```python
from build123d import *

# Parameters (mm, degrees)
SKETCH2_R         = 0.8
SKETCH4_R         = 0.9
EXTRUDE1_DEPTH    = 6
SKETCH5_OUTSIDE_W = 12.282
SKETCH5_OUTSIDE_H = 20.656
SKETCH5_OUTSIDE_R = 0.75
EXTRUDE3_DEPTH    = 11


with BuildPart() as part:
    # Sweep1: sweep along a path in Sketch1
    with BuildLine(Plane(origin=(0, 0, 0), x_dir=(0, 0, -1), z_dir=(1, 0, 0))) as sweep1_path:
        Line((-7.5, 0), (-7.5, 35))
        ThreePointArc((-7.5, 35), (-8.042543867, 36.720729309), (-9.47393957, 37.819077862))
        Line((-9.47393957, 37.819077862), (-16.5, 40.376354723))
    # Sketch2 → Sweep1 (sweep)
    with BuildSketch(Plane(origin=(0, 0, 0), x_dir=(1, 0, 0), z_dir=(0, 1, 0))):
        with Locations((0, -7.5)):
            Circle(SKETCH2_R)
    sweep(path=sweep1_path.line)

    # Sketch4 → Extrude1 (add)
    with BuildSketch(Plane(origin=(0, 0, 0), x_dir=(1, 0, 0), z_dir=(0, 1, 0))):
        with Locations((0, -7.5)):
            Circle(SKETCH4_R)
    extrude(amount=EXTRUDE1_DEPTH)

    # Sketch5 outside → Extrude3 (cut)
    with BuildSketch(Plane(origin=(0, 19, 0), x_dir=(-1, 0, 0), z_dir=(0, 1, 0))):
        with Locations((0, 11.687)):
            Rectangle(SKETCH5_OUTSIDE_W, SKETCH5_OUTSIDE_H)
        with Locations((0, 7.5)):
            Circle(SKETCH5_OUTSIDE_R, mode=Mode.SUBTRACT)
    extrude(amount=EXTRUDE3_DEPTH, mode=Mode.SUBTRACT)


solid = part.part
```
The listing builds one solid part. Answer for the finished solid, in the listing's coordinates (mm). A direction names the side the tool comes from. Give positions to 0.01 mm unless a question says otherwise; leave off trailing zeros. Loops run counter-clockwise (first coordinate to the right, second up) from the corner with the lowest first, then second, coordinate; pieces in that order, holes last. Notation, with made-up numbers: M 8.5,73.5 L 48.5,73.5 A27 ccw 48.5,102.5 Z; hole C -6.5,-21 d10. An arc over 180 degrees is marked long. One line per item, written item: value.
1. Section B-B on y = 6.5 is taken. Determine the outline of the cut face in (x, z).
Found:
outline: C 0,7.5 d1.6
2. Section A-A on x = 0 is taken. Determine the outline of the cut face in (y, z), plus the area to 3 significant figures.
Found:
outline: M 0,6.6 L 6,6.6 L 6,6.7 L 19,6.7 L 19,6.75 L 30,6.75 L 30,6.7 L 35,6.7 A3.8 ccw 38.57,9.2 L 41.13,16.23 L 39.62,16.77 L 37.07,9.75 A2.2 cw 35,8.3 L 30,8.3 L 30,8.25 L 19,8.25 L 19,8.3 L 6,8.3 L 6,8.4 L 0,8.4 Z
area: 73.9 mm^2
3. Find the intervals of material crossed by probe 1 along Z at (x, y) = (0.1, 24.5); probe 2 along Z at (x, y) = (0.4, 5); probe 3 along Y at (x, z) = (0, 11.5), in increasing order.
Found:
probe 1: 6.76 to 8.24
probe 2: 6.69 to 8.31
probe 3: 37.71 to 39.41
4. For a pull along Y with two mould halves and no side action, classify faces 3 (the face through (-0.104, 12.591, 6.707)), 4 (the face through (0.55, 24.42, 8.01)), 5 (the face through (-0.12, 2.96, 6.61)), 6 (the face through (0, 0, 7)) as pulls with the +Y half, pulls with the -Y half, needs draft (parallel to the pull), parting line crosses it, or undercut.
Found:
face 3: undercut
face 4: undercut
face 5: needs draft
face 6: pulls with the -Y half
5. Each of these flat-tipped pins is pushed along its axis until it touches: P1, Ø0.5, axis at x = 0, z = 7.5, coming from the +Y side; P2, Ø1, axis at x = 0, z = 8, coming from the +Y side. Where does it stop, or does it pass through?
Found:
P1: y = 37.62
P2: y = 38.23
6. For faces 1 (the face through (-0.104, 32.535, 6.707)), 2 (the face through (-0.011, 40.366, 16.504)), determine the directions among +Z, -Z, +X, -X, +Y, -Y from which every point of the face is accessible in a straight line to the end or side of a thin tool.
Found:
face 1: none
face 2: +Z, +X, -X, +Y
